```python
from build123d import *

# Parameters (mm, degrees)
BOSS_EXTRUDE2_DEPTH = 12.7
SKETCH2_W           = 50.8
SKETCH2_H           = 19.05
CUT_EXTRUDE1_DEPTH  = 256.917605149


with BuildPart() as part:
    # Sketch1 → Boss-Extrude2 (new, symmetric)
    with BuildSketch(Plane.XY):
        Polygon((-25.4, -127), (-25.4, -76.2), (25.4, -76.2), (25.4, -127), (28.575, -127), (28.575, 127), (-28.575, 127), (-28.575, -127), align=None)
    extrude(amount=BOSS_EXTRUDE2_DEPTH, both=True)

    # Sketch2 → Cut-Extrude1 (cut, through all)
    with BuildSketch(Plane(origin=(0, 127, 0), x_dir=(1, 0, 0), z_dir=(0, 1, 0))):
        Rectangle(SKETCH2_W, SKETCH2_H)
    extrude(amount=-CUT_EXTRUDE1_DEPTH, mode=Mode.SUBTRACT)


solid = part.part
```
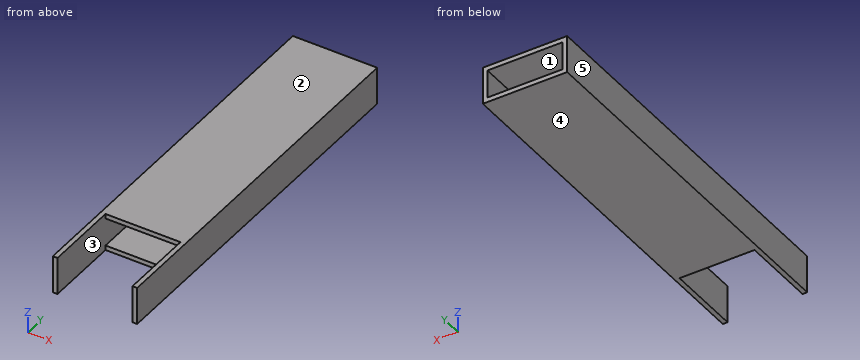
Source: CAD feature listing. Evaluate the final solid. Frame: model axes, mm. Face numbers are marked on the shaded views. A direction names the side the tool comes from. Round coordinates to 2 decimals unless told otherwise and drop trailing zeros. Loops run counter-clockwise (first coordinate to the right, second up) from the corner with the lowest first, then second, coordinate; pieces in that order, holes last. Notation, with made-up numbers: M -10.75,-29.5 L -6.75,-29.5 A23 cw -6.75,-14.5 Z; hole C -25,-9 d9. An arc over 180 degrees is marked long. Use a Markdown table: item, result. Add a question column.
1. Line query: line 1 (Z direction, x = 3, y = 69) (3 decimals); line 2 (X direction, y = 52.5, z = -5.5) (3 decimals); line 3 (Y direction, x = 25, z = 10.5). Output: solid intervals per line, ascending.
2. Contact query for a flat-ended pin moving along its axis: P1, Ø1, axis at x = 6, z = 12, coming from the -Y side. Output: stop coordinate, or through.
3. Mould query, pull axis Z, two halves, no side actions, for the marked faces 3, 4 and 5. Classes: pulls with the +Z half, pulls with the -Z half, needs draft (parallel to the pull), parting line crosses it, or undercut.
4. Section query A-A on z = 3. Return the cut outline in (x, y) (3 decimals).
5. Reachability of the marked faces 1 and 2 from +Z, -Z, +X, -X, +Y, -Y: full face, straight path, thin tool, end or side. Return the list, or none.
6. Section query C-C on y = -66.5. Return the cut outline in (x, z) (3 decimals).
7. Section query B-B on x = 5.5. Return the cut outline in (y, z) (3 decimals), then the cut area to 3 significant figures.
Reported:
| question | item | result |
|---|---|---|
| 1 | line 1 | z = -12.7 to -9.525, 9.525 to 12.7 |
| 1 | line 2 | x = -28.575 to -25.4, 25.4 to 28.575 |
| 1 | line 3 | y = -76.2 to 127 |
| 2 | P1 | stops at y = -76.2 |
| 3 | face 3 | undercut |
| 3 | face 4 | pulls with the -Z half |
| 3 | face 5 | needs draft |
| 4 | outline | M -28.575,-127 L -25.4,-127 L -25.4,127 L -28.575,127 Z; M 25.4,-127 L 28.575,-127 L 28.575,127 L 25.4,127 Z |
| 5 | face 1 | +Y, -Y |
| 5 | face 2 | +Z, +X, -X, +Y, -Y |
| 6 | outline | M -28.575,-12.7 L 28.575,-12.7 L 28.575,12.7 L -28.575,12.7 Z; hole M -25.4,-9.525 L 25.4,-9.525 L 25.4,9.525 L -25.4,9.525 Z |
| 7 | outline | M -76.2,-12.7 L 127,-12.7 L 127,-9.525 L -76.2,-9.525 Z; M -76.2,9.525 L 127,9.525 L 127,12.7 L -76.2,12.7 Z |
| 7 | area | 1,290 mm² |
